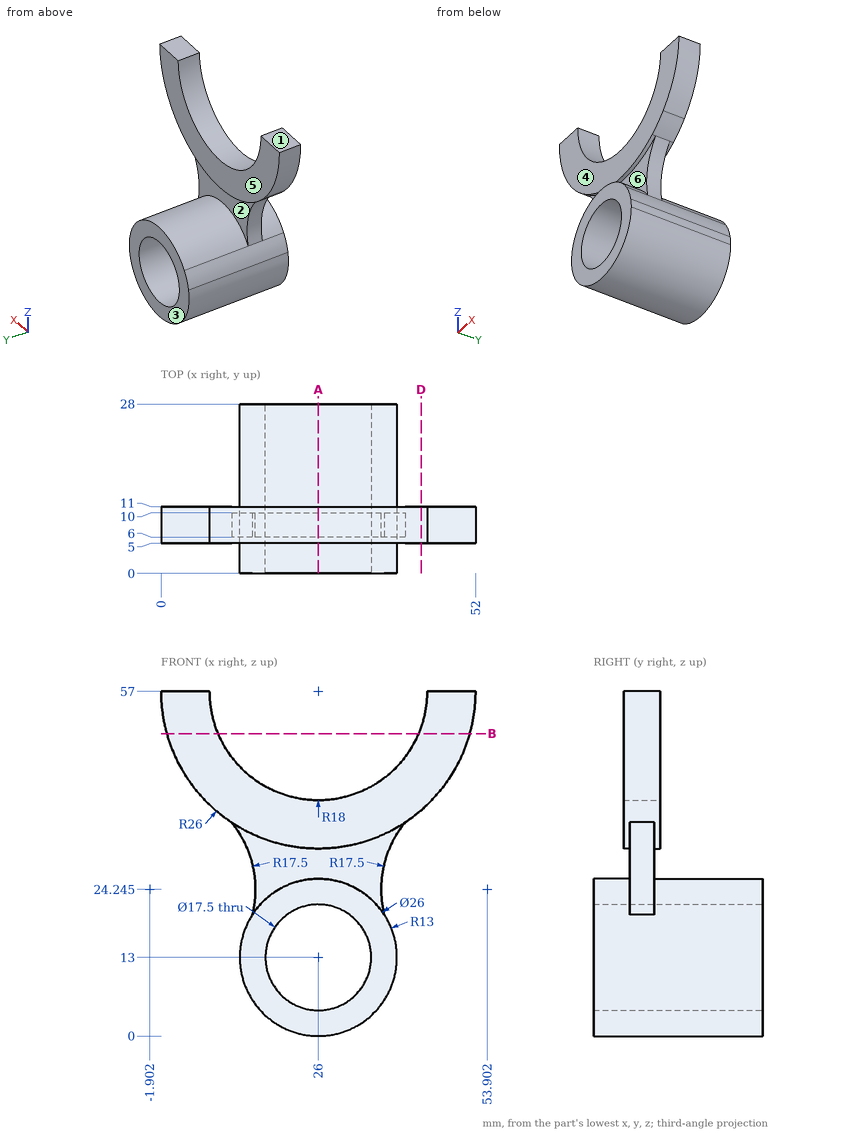
The drawing under review shows one solid part. Ordinate dimensions are in mm from its lowest x, y, z. A direction names the side the tool comes from. Round coordinates to 2 decimals unless told otherwise and drop trailing zeros. Loops run counter-clockwise (first coordinate to the right, second up) from the corner with the lowest first, then second, coordinate; pieces in that order, holes last. Notation, with made-up numbers: (34, 69) - (64, 69) arc R12 cw to (64, 90) - close; hole circle Ø5 at (81, 50). An arc over 180 degrees is marked (long way). One line per question, with ' | ' between items.
1. For the marked faces 4, 5 and 6, list the 3-axis set-ups (+Z, -Z, +X, -X, +Y, -Y) from which the entire face can be reached by the end or side of a thin tool; tool diameter is ignored.
Results are:
face 4: +Z, +X, -X, -Y | face 5: +Z, +X, -X, +Y | face 6: -Y
2. Clearance check with flat-ended pins moving along their axes: P1, Ø7.5, axis at x = 27.5, z = 29.5, coming from the +Y side; P2, Ø5, axis at x = 36, y = 4, coming from the +Z side; P3, Ø5, axis at x = 45, y = 11, coming from the -Z side (1 decimal); P4, Ø3, axis at x = 21.5, y = 5.5, coming from the -Z side. State where each tip first meets the part, or that it passes through.
Results are:
P1: stops at y = 28 | P2: stops at z = 43.85 | P3: stops at z = 36.9 | P4: stops at z = 0.35
3. For L1, parallel to Z at x = 26, y = 10.75; L2, parallel to Z at x = 26, y = 19.5; L3, parallel to X at y = 17.75, z = 13, list the stretches that pass through material, from the lowest coordinate up. Write a range as [from, to].
Results are:
L1: z = [0, 4.25], [21.75, 26], [31, 39] | L2: z = [0, 4.25], [21.75, 26] | L3: x = [13, 17.25], [34.75, 39]
4. Draft analysis for pull direction Z (two halves, no side actions). For the marked faces 1, 2 and 3, state which applies: released by +Z, released by -Z, zero draft, split by the parting line, or undercut.
Results are:
face 1: released by +Z | face 2: undercut | face 3: zero draft
5. We need section B-B, the plane z = 50. State the section outline as (x, y) points.
Results are:
outline: (0.96, 5) - (9.42, 5) - (9.42, 11) - (0.96, 11) - close; (42.58, 5) - (51.04, 5) - (51.04, 11) - (42.58, 11) - close
6. We need section A-A, the plane x = 26. State the section outline as (y, z) points, and give its area (3 significant figures).
Results are:
outline: (0, 0) - (28, 0) - (28, 4.25) - (0, 4.25) - close; (0, 21.75) - (28, 21.75) - (28, 26) - (10, 26) - (10, 31) - (11, 31) - (11, 39) - (5, 39) - (5, 31) - (6, 31) - (6, 26) - (0, 26) - close | area: 306 mm²
7. We need section D-D, the plane x = 43. State the section outline as (y, z) points.
Results are:
outline: (5, 37.33) - (11, 37.33) - (11, 51.08) - (5, 51.08) - close
